Geometry: see drawing. Coordinates: mm, zero at the bounding-box minimum. A direction names the side the tool comes from. Coordinates: 2 decimals unless noted, no trailing zeros. Order: outer loops, then holes, each group sorted by start corner. A loop starts at its lowest first (then second) coordinate and runs counter-clockwise, first axis right, second up. Notation, with made-up numbers: M 48.5,83 L 102.5,83 A13 cw 102.5,98 Z; hole C 70.25,58.25 d11. An arc over 180 degrees is marked long. Answer in a Markdown table with one row per item.
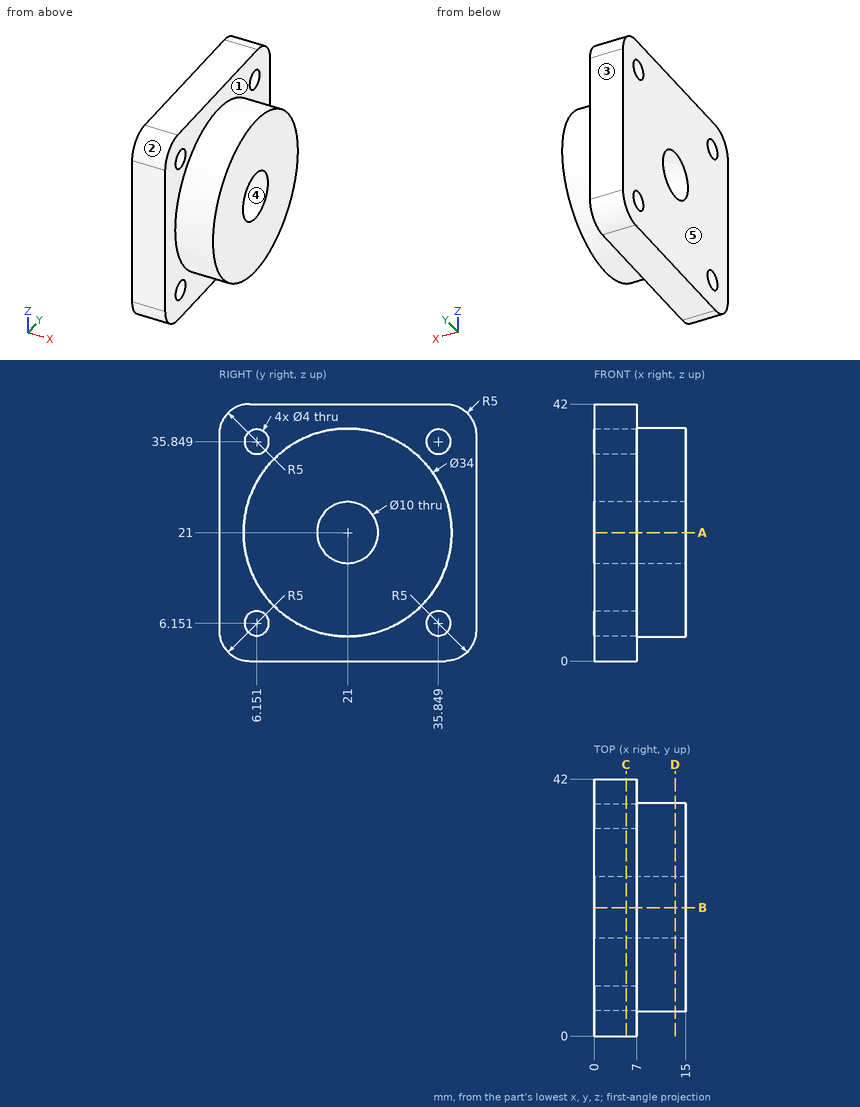
1) Contact query for flat-ended pins moving along their axis: pin 1 (3.5 mm diameter, centred on y = 35.85, z = 6.15, fed in from +X); pin 2 (8 mm diameter, centred on x = 11.5, z = 19, fed in from -Y); pin 3 (5 mm diameter, centred on y = 35.85, z = 35.85, fed in from +X). Output: stop coordinate, or through.
Resolved:
| item | result |
|---|---|
| pin 1 | passes through |
| pin 2 | stops at y = 4 |
| pin 3 | stops at x = 7 |
2) Cut plane D-D, the plane x = 13.25. Output: boundary loops of the cut face in (y, z).
Resolved:
| item | result |
|---|---|
| outline | C 21,21 d34; hole C 21,21 d10 |
3) Material intervals for probe 1 along Y at (x, z) = (3, 36) (1 decimal); probe 2 along Z at (x, y) = (2.25, 5) (1 decimal); probe 3 along X at (y, z) = (40, 33), sorted ascending.
Resolved:
| item | result |
|---|---|
| probe 1 | y = 0 to 4.2, 8.1 to 33.9, 37.8 to 42 |
| probe 2 | z = 0 to 4.5, 7.8 to 34.2, 37.5 to 42 |
| probe 3 | x = 0 to 7 |
4) Reachability of the marked faces 1 and 2 from +Z, -Z, +X, -X, +Y, -Y: full face, straight path, thin tool, end or side. Return the list, or none.
Resolved:
| item | result |
|---|---|
| face 1 | +X |
| face 2 | +Z, +X, -X, -Y |
5) Mould query, pull axis Y, two halves, no side actions, for the marked faces 3, 4 and 5. Classes: +Y half, -Y half, draft (parallel to the pull), parting line (faces both ways), or undercut.
Resolved:
| item | result |
|---|---|
| face 3 | +Y half |
| face 4 | undercut |
| face 5 | draft |
6) Cut plane A-A, the plane z = 21. Output: boundary loops of the cut face in (x, y), and give its area (3 significant figures).
Resolved:
| item | result |
|---|---|
| outline | M 0,0 L 7,0 L 7,4 L 15,4 L 15,16 L 0,16 Z; M 0,26 L 15,26 L 15,38 L 7,38 L 7,42 L 0,42 Z |
| area | 416 mm2 |
7) Cut plane C-C, the plane x = 5.25. Output: boundary loops of the cut face in (y, z).
Resolved:
| item | result |
|---|---|
| outline | M 0,5 A5 ccw 5,0 L 37,0 A5 ccw 42,5 L 42,37 A5 ccw 37,42 L 5,42 A5 ccw 0,37 Z; hole C 6.15,6.15 d4; hole C 6.15,35.85 d4; hole C 21,21 d10; hole C 35.85,6.15 d4; hole C 35.85,35.85 d4 |
